from build123d import *

# Parameters (mm, degrees)
SKETCH1_W           = 42.62295082
SKETCH1_H           = 50
SKETCH1_R           = 2.677018134
BOSS_EXTRUDE1_DEPTH = 16
SKETCH2_R           = 11
CUT_EXTRUDE2_DEPTH  = 11
SKETCH3_R           = 1.75
CUT_EXTRUDE3_DEPTH  = 10
SKETCH6_W           = 9.034037672
SKETCH6_H           = 2.387531408
CUT_EXTRUDE5_DEPTH  = 20
CUT_EXTRUDE6_START  = -5
CUT_EXTRUDE6_DEPTH  = 32.540101042


with BuildPart() as part:
    # Sketch1 → Boss-Extrude1 (new body)
    with BuildSketch(Plane.XY):
        Rectangle(SKETCH1_W, SKETCH1_H)
        with Locations((-13, -15.25)):
            Circle(SKETCH1_R, mode=Mode.SUBTRACT)
        with Locations(Location((13, -15.25, 0), (0, 0, 180))):
            Circle(SKETCH1_R, mode=Mode.SUBTRACT)
        with Locations((13, 15.25)):
            Circle(SKETCH1_R, mode=Mode.SUBTRACT)
        with Locations(Location((-13, 15.25, 0), (0, 0, 180))):
            Circle(SKETCH1_R, mode=Mode.SUBTRACT)
    extrude(amount=BOSS_EXTRUDE1_DEPTH)

    # Sketch2 → Cut-Extrude2 (cut)
    with BuildSketch(Plane.XY):
        Circle(SKETCH2_R)
    extrude(amount=CUT_EXTRUDE2_DEPTH, mode=Mode.SUBTRACT)

    # Sketch3 → Cut-Extrude3 (cut)
    with BuildSketch(Plane(origin=(0, 0, 0), x_dir=(-1, 0, 0), z_dir=(0, 0, -1))):
        with Locations((-15, 0)):
            Circle(SKETCH3_R)
        with Locations(Location((15, 0, 0), (0, 0, 180))):
            Circle(SKETCH3_R)
    extrude(amount=-CUT_EXTRUDE3_DEPTH, mode=Mode.SUBTRACT)

    # Sketch6 → Cut-Extrude5 (cut)
    with BuildSketch(Plane.XZ.offset(25)):
        with Locations((0, 12.193765704)):
            Rectangle(SKETCH6_W, SKETCH6_H)
    extrude(amount=-CUT_EXTRUDE5_DEPTH, mode=Mode.SUBTRACT)

    # Sketch9 → Cut-Extrude6 (cut, through all)
    with BuildSketch(Plane(origin=(0, 0, 0), x_dir=(-1, 0, 0), z_dir=(0, 0, -1)).offset(CUT_EXTRUDE6_START)):
        Polygon((-15, 3.175426481), (-17.75, 1.58771324), (-17.75, -1.58771324), (-15, -3.175426481), (-12.25, -1.58771324), (-12.25, 1.58771324), align=None)
        Polygon((12.25, 1.58771324), (15, 3.175426481), (17.75, 1.58771324), (17.75, -1.58771324), (15, -3.175426481), (12.25, -1.58771324), align=None)
    extrude(amount=-CUT_EXTRUDE6_DEPTH, mode=Mode.SUBTRACT)


solid = part.part
Verification items for the finished model (mm, model axes). A direction names the side the tool comes from. Round coordinates to 2 decimals unless told otherwise and drop trailing zeros. Write each loop counter-clockwise with the first axis right and the second up, starting at its lowest first coordinate (ties: lowest second). Pieces come first, ordered by that corner, then holes.
(1) Material ranges on line 1 (Y direction, x = -11.5, z = 5.25); line 2 (Y direction, x = 13.5, z = 6.25); line 3 (X direction, y = -0.5, z = 13.75), recorded low to high.
Returned:
line 1: y = -25 to -17.47, -13.03 to 13.03, 17.47 to 25
line 2: y = -25 to -17.88, -12.62 to -2.31, 2.31 to 12.62, 17.88 to 25
line 3: x = -21.31 to -17.75, -12.25 to 12.25, 17.75 to 21.31
(2) Section check C-C (y = -14). Enter the section's corners in (x, z).
Returned:
outline: (-21.31, 0) - (-15.37, 0) - (-15.37, 16) - (-21.31, 16) - close; (-10.63, 0) - (10.63, 0) - (10.63, 16) - (-10.63, 16) - close; (15.37, 0) - (21.31, 0) - (21.31, 16) - (15.37, 16) - close; hole (-4.52, 11) - (4.52, 11) - (4.52, 13.39) - (-4.52, 13.39) - close
(3) Access from +Z, -Z, +X, -X, +Y, -Y to the whole of each face (thin tool, end or side, straight path). Record for faces 1 (the flat face through (16.394, -2.37, 10.423)), 2 (the flat face through (4.517, -15, 12)), 3 (the flat face through (0, -5, 12)).
Returned:
face 1: +Z
face 2: -Y
face 3: -Z, -Y
(4) Mould release check, pull along Z, two halves, no side actions. Record for faces 4 (the flat face through (16.3, -1.4, 5)), 5 (the cylindrical face through (12.42, 12.637, 7.888)), 6 (the flat face through (-4.517, -15, 12)): pulls with the +Z half, pulls with the -Z half, needs draft (parallel to the pull), parting line crosses it, or undercut.
Returned:
face 4: pulls with the +Z half
face 5: needs draft
face 6: undercut
(5) Depth check by flat-ended pin: pin 1 Ø2.5 at (x, y) = (1.5, -14) entering from -Z; pin 2 Ø0.7 at (x, z) = (-2, 12) entering from -Y. Enter the tip coordinate at first touch or a pass-through.
Returned:
pin 1: stops at z = 0
pin 2: stops at y = -5
(6) Section check B-B (y = 0). Enter the section's corners in (x, z).
Returned:
outline: (-21.31, 0) - (-16.75, 0) - (-16.75, 5) - (-17.75, 5) - (-17.75, 16) - (-21.31, 16) - close; (-13.25, 0) - (-11, 0) - (-11, 11) - (11, 11) - (11, 0) - (13.25, 0) - (13.25, 5) - (12.25, 5) - (12.25, 16) - (-12.25, 16) - (-12.25, 5) - (-13.25, 5) - close; (16.75, 0) - (21.31, 0) - (21.31, 16) - (17.75, 16) - (17.75, 5) - (16.75, 5) - close
(7) Section check A-A (x = 0). Enter the section's corners in (y, z).
Returned:
outline: (-25, 0) - (-11, 0) - (-11, 11) - (-25, 11) - close; (-25, 13.39) - (-5, 13.39) - (-5, 11) - (11, 11) - (11, 0) - (25, 0) - (25, 16) - (-25, 16) - close
(8) Section check D-D (z = 8.75). Enter the section's corners in (x, y), plus the area to 3 significant figures.
Returned:
outline: (-21.31, -25) - (21.31, -25) - (21.31, 25) - (-21.31, 25) - close; hole (-17.75, -1.59) - (-15, -3.18) - (-12.25, -1.59) - (-12.25, 1.59) - (-15, 3.18) - (-17.75, 1.59) - close; hole circle Ø5.35 at (-13, -15.25); hole circle Ø5.35 at (-13, 15.25); hole circle Ø22 at (0, 0); hole circle Ø5.35 at (13, -15.25); hole circle Ø5.35 at (13, 15.25); hole (12.25, -1.59) - (15, -3.18) - (17.75, -1.59) - (17.75, 1.59) - (15, 3.18) - (12.25, 1.59) - close
area: 1,610 mm2
